The drawing under review shows one solid part. Ordinate dimensions are in mm from its lowest x, y, z. A direction names the side the tool comes from. Coordinates: 2 decimals unless noted, no trailing zeros. Order: outer loops, then holes, each group sorted by start corner. A loop starts at its lowest first (then second) coordinate and runs counter-clockwise, first axis right, second up. Notation, with made-up numbers: (-24.75, -21.75) -> (-12.75, -21.75) arc R11 ccw to (-12.75, -0.75) -> close; hole circle Ø2 at (-22.75, 49.5). An arc over 180 degrees is marked (long way). Put each result on its own line as item: value.
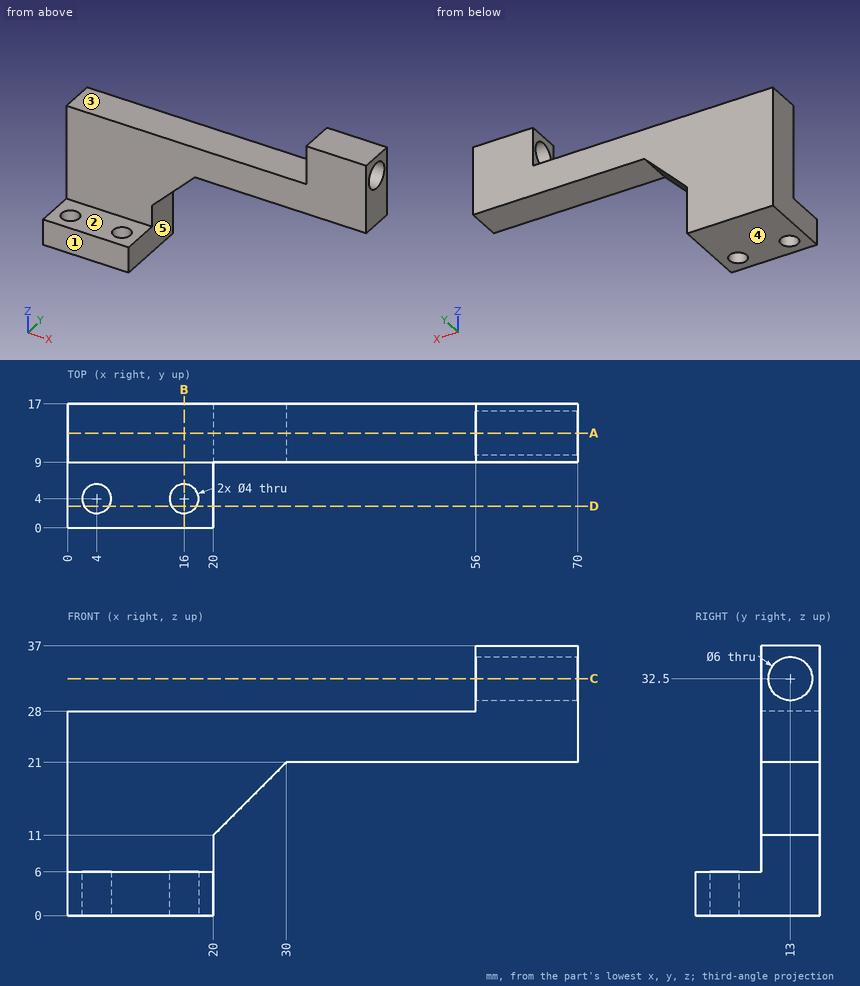
Item 1: For line 1 (Y direction, x = 4, z = 1.8); line 2 (Y direction, x = 55.5, z = 26); line 3 (Y direction, x = 63, z = 32.5), list the stretches that pass through material, from the lowest coordinate up. Write a range as from..to.
Answers below:
line 1: 0..2, 6..17
line 2: 9..17
line 3: 9..10, 16..17
Item 2: For pin 1 Ø6 at (x, z) = (25.5, 13.5) entering from -Y; pin 2 Ø9 at (y, z) = (10.5, 8) entering from +X; pin 3 Ø2.5 at (x, y) = (38.5, 14) entering from +Z, all flat-tipped, find the tip position at first contact; note any pin that passes through.
Answers below:
pin 1: y = 9
pin 2: x = 21.5
pin 3: z = 28
Item 3: Consider section C-C on z = 32.5. Write out the cut boundary in (x, y).
Answers below:
outline: (56, 9) -> (70, 9) -> (70, 10) -> (56, 10) -> close; (56, 16) -> (70, 16) -> (70, 17) -> (56, 17) -> close
Item 4: Consider section A-A on y = 13. Write out the cut boundary in (x, z).
Answers below:
outline: (0, 0) -> (20, 0) -> (20, 11) -> (30, 21) -> (70, 21) -> (70, 29.5) -> (56, 29.5) -> (56, 28) -> (0, 28) -> close; (56, 35.5) -> (70, 35.5) -> (70, 37) -> (56, 37) -> close
Item 5: Consider section B-B on x = 16. Write out the cut boundary in (y, z).
Answers below:
outline: (0, 0) -> (2, 0) -> (2, 6) -> (0, 6) -> close; (6, 0) -> (17, 0) -> (17, 28) -> (9, 28) -> (9, 6) -> (6, 6) -> close
Item 6: Consider section D-D on y = 3. Write out the cut boundary in (x, z), and give its area (3 significant figures).
Answers below:
outline: (0, 0) -> (2.27, 0) -> (2.27, 6) -> (0, 6) -> close; (5.73, 0) -> (14.27, 0) -> (14.27, 6) -> (5.73, 6) -> close; (17.73, 0) -> (20, 0) -> (20, 6) -> (17.73, 6) -> close
area: 78.4 mm^2
Item 7: For the marked faces 1, 2, 3, 4 and 5, list the 3-axis set-ups (+Z, -Z, +X, -X, +Y, -Y) from which the entire face can be reached by the end or side of a thin tool; tool diameter is ignored.
Answers below:
face 1: +Z, -Z, +X, -X, -Y
face 2: +Z, +X, -X, -Y
face 3: +Z, -X, +Y, -Y
face 4: -Z, +X, -X, +Y, -Y
face 5: -Z, +X, +Y, -Y
